Read the model definition and answer for the solid it produces. Units are mm, in the model's axes. Give positions to 0.01 mm unless a question says otherwise; leave off trailing zeros. Order: outer loops, then holes, each group sorted by start corner. A loop starts at its lowest first (then second) coordinate and runs counter-clockwise, first axis right, second up.
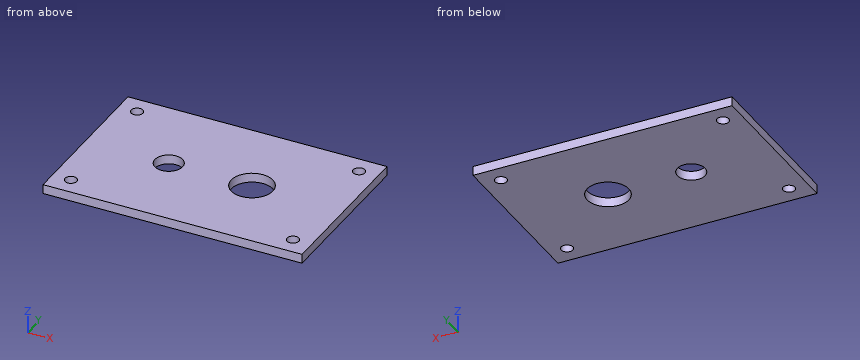
```python
from build123d import *

# Parameters (mm, degrees)
SKETCH1_W           = 177.8
SKETCH1_H           = 114.3
SKETCH1_R           = 14.2875
SKETCH1_R_2         = 9.525
SKETCH1_R_3         = 4.064
BOSS_EXTRUDE1_DEPTH = 3.175


with BuildPart() as part:
    # Sketch1 → Boss-Extrude1 (new, symmetric)
    with BuildSketch(Plane.XY):
        Rectangle(SKETCH1_W, SKETCH1_H)
        with Locations((25.4, 0)):
            Circle(SKETCH1_R, mode=Mode.SUBTRACT)
        with Locations((-31.75, 0)):
            Circle(SKETCH1_R_2, mode=Mode.SUBTRACT)
        with Locations((-76.2, 44.45)):
            Circle(SKETCH1_R_3, mode=Mode.SUBTRACT)
        with Locations(Location((-76.2, -44.45, 0), (0, 0, 180))):
            Circle(SKETCH1_R_3, mode=Mode.SUBTRACT)
        with Locations(Location((76.2, 44.45, 0), (0, 0, 180))):
            Circle(SKETCH1_R_3, mode=Mode.SUBTRACT)
        with Locations((76.2, -44.45)):
            Circle(SKETCH1_R_3, mode=Mode.SUBTRACT)
    extrude(amount=BOSS_EXTRUDE1_DEPTH, both=True)


solid = part.part
```
1) The part is cut by section A-A on y = -44.45. Determine the outline of the cut face in (x, z) (3 decimals).
Final values:
outline: (-88.9, -3.175) - (-80.264, -3.175) - (-80.264, 3.175) - (-88.9, 3.175) - close; (-72.136, -3.175) - (72.136, -3.175) - (72.136, 3.175) - (-72.136, 3.175) - close; (80.264, -3.175) - (88.9, -3.175) - (88.9, 3.175) - (80.264, 3.175) - close
2) Consider L1, parallel to X at y = -7, z = -0.75; L2, parallel to Y at x = -31.75, z = 0.75 (3 decimals); L3, parallel to X at y = 3.5, z = -0.25. Determine where each line is inside the solid, lowest interval first.
Final values:
L1: x = -88.9 to -38.21, -25.29 to 12.94, 37.86 to 88.9
L2: y = -57.15 to -9.525, 9.525 to 57.15
L3: x = -88.9 to -40.61, -22.89 to 11.55, 39.25 to 88.9
3) The part is cut by section B-B on x = -76.2. Determine the outline of the cut face in (y, z) (3 decimals), and give its area (3 significant figures).
Final values:
outline: (-57.15, -3.175) - (-48.514, -3.175) - (-48.514, 3.175) - (-57.15, 3.175) - close; (-40.386, -3.175) - (40.386, -3.175) - (40.386, 3.175) - (-40.386, 3.175) - close; (48.514, -3.175) - (57.15, -3.175) - (57.15, 3.175) - (48.514, 3.175) - close
area: 623 mm2
4) The part is cut by section C-C on z = 0. Count the separate pieces of the cut face and the enclosed holes in it, and give its area (3 significant figures).
Final values:
separate pieces: 1
enclosed holes: 6
area: 19,200 mm2
5) The part is cut by section D-D on x = -32. Determine the outline of the cut face in (y, z) (3 decimals), and give its area (3 significant figures).
Final values:
outline: (-57.15, -3.175) - (-9.522, -3.175) - (-9.522, 3.175) - (-57.15, 3.175) - close; (9.522, -3.175) - (57.15, -3.175) - (57.15, 3.175) - (9.522, 3.175) - close
area: 605 mm2
